Work out the finished part from the listing and answer in its coordinate system (mm). A direction names the side the tool comes from. Coordinates: 2 decimals unless noted, no trailing zeros. Loops run counter-clockwise (first coordinate to the right, second up) from the corner with the lowest first, then second, coordinate; pieces in that order, holes last. Notation, with made-up numbers: (64.5, 16) -> (73.5, 16) arc R24 cw to (73.5, 32) -> close; hole circle Ø8 at (17.25, 89). An arc over 180 degrees is marked (long way). Answer as CSV lines item,"result".
```python
from build123d import *

# Parameters (mm, degrees)
SALIENTE_EXTRUIR1_DEPTH = 29
VACIADO3_T              = -1.5


with BuildPart() as part:
    # Croquis1 → Saliente-Extruir1 (new, symmetric)
    with BuildSketch(Plane.XY):
        with BuildLine():
            Line((-288.592886812, -13.410938253), (286.407113188, -13.410938253))
            ThreePointArc((286.407113188, -13.410938253), (302.048282251, -1.185571473), (288.592886812, 13.410938253))
            Line((288.592886812, 13.410938253), (-286.407113188, 13.410938253))
            ThreePointArc((-286.407113188, 13.410938253), (-299.862508627, 1.00744798), (-288.592886812, -13.410938253))
        make_face()
    extrude(amount=SALIENTE_EXTRUIR1_DEPTH, both=True)

    # Vaciado3
    vaciado3_openings = [part.faces().sort_by_distance(p)[0] for p in [
        (1.102229912, -0.003188018, 29),
        (1.102229912, -0.003188018, -29),
    ]]
    offset(amount=VACIADO3_T, openings=vaciado3_openings, kind=Kind.INTERSECTION)


solid = part.part
```
(1) A cutting plane is placed at B-B, the plane y = 2. Write down the section's boundary in (x, z).
Computed values:
outline,"(-299.74, -29) -> (-298.22, -29) -> (-298.22, 29) -> (-299.74, 29) -> close; (300.41, -29) -> (301.93, -29) -> (301.93, 29) -> (300.41, 29) -> close"
(2) For a pull along X with two mould halves and no side action, classify faces 3 (the face through (5, 11.911, 0)), 4 (the face through (-299.837, 1.288, 0.406)), 5 (the face through (-5, -13.411, 0)) as pulls with the +X half, pulls with the -X half, needs draft (parallel to the pull), parting line crosses it, or undercut.
Computed values:
face 3,"undercut"
face 4,"pulls with the -X half"
face 5,"needs draft"
(3) Flat-ended cylindrical pins translate along their axes: pin 1 Ø8 at (y, z) = (-7.5, 19.5) entering from -X; pin 2 Ø4 at (x, z) = (191, 8.5) entering from -Y; pin 3 Ø6 at (y, z) = (10.5, 7) entering from -X. Find the tip coordinate at first contact, or state that the pin passes through.
Computed values:
pin 1,"x = -299.47"
pin 2,"y = -13.41"
pin 3,"x = -297.57"
(4) A cutting plane is placed at C-C, the plane z = 1.5. Write down the section's boundary in (x, y), and give its area (3 significant figures).
Computed values:
outline,"(-288.59, -13.41) -> (286.41, -13.41) arc R13.5 ccw (long way) to (288.59, 13.41) -> (-286.41, 13.41) arc R13.5 ccw to start; hole (-288.47, -11.91) -> (286.53, -11.91) arc R12 ccw (long way) to (288.59, 11.91) -> (-286.41, 11.91) arc R12 ccw to start"
area,"1,850 mm2"
(5) A cutting plane is placed at A-A, the plane x = 172.5. Write down the section's boundary in (y, z), and give its area (3 significant figures).
Computed values:
outline,"(-13.41, -29) -> (-11.91, -29) -> (-11.91, 29) -> (-13.41, 29) -> close; (11.91, -29) -> (13.41, -29) -> (13.41, 29) -> (11.91, 29) -> close"
area,"174 mm2"
(6) Consider line 1 along Y through (x, z) = (13, -8); line 2 along X through (y, z) = (0.5, 2); line 3 along X through (y, z) = (-5.5, -13.5). Determine where each line is inside the solid, lowest interval first.
Computed values:
line 1,"-13.41 to -11.91, 11.91 to 13.41"
line 2,"-299.89 to -298.39, 300.58 to 302.08"
line 3,"-298.78 to -297.12, 299.3 to 300.96"
(7) Which of the six approach directions +Z, -Z, +X, -X, +Y, -Y give full straight-line access (tool end or side, diameter ignored) to faces 1 (the face through (0, -13, 29)), 2 (the face through (-298.34, 1.19, 0.41))?
Computed values:
face 1,"+Z, +X, -X, +Y, -Y"
face 2,"+Z, -Z"
